Can you work these out from the model? Positions are in its coordinate system, mm. Face numbers are marked on the shaded views. Round coordinates to 2 decimals unless told otherwise and drop trailing zeros. Write each loop counter-clockwise with the first axis right and the second up, starting at its lowest first coordinate (ties: lowest second). Pieces come first, ordered by that corner, then holes.
Q1. We'd pull the mould along Z, two halves only. Please class the marked faces 1, 2, 3 and 4: +Z half, -Z half, draft (parallel to the pull), parting line (faces both ways), or undercut.
Q2. I'm going to push flat-ended pins straight in: pin 1 Ø5 at (y, z) = (-7, -2) entering from -X; pin 2 Ø5 at (x, z) = (13.5, 0) entering from +Y; pin 3 Ø1.5 at (y, z) = (-1.5, 9) entering from -X; pin 4 Ø1 at (x, y) = (-11.5, -4) entering from +Z. Where does each tip first touch, or does it pass through?
Q3. If we section it at B-B (y = -9.5): Please give me the cut outline in (x, z), plus the area to 3 significant figures.
Q4. If we section it at A-A (x = -5.5): Please give me the cut outline in (y, z).
Q5. Please list where these lines run through material, in increasing order: line 1 along Z through (x, y) = (13.5, -4); line 2 along Z through (x, y) = (-13, -10.5); line 3 along X through (y, z) = (-11, 1.5).
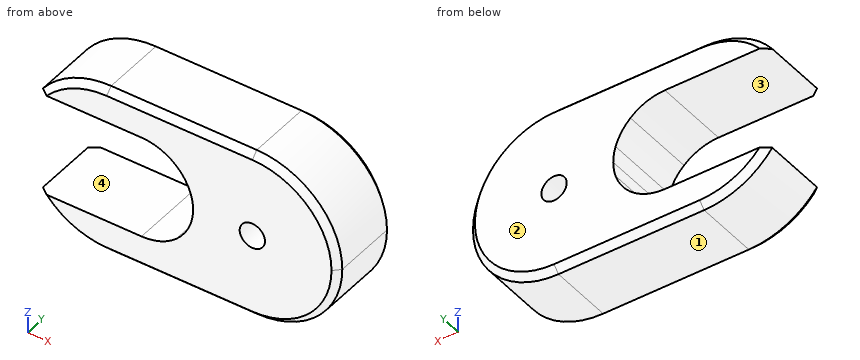
from build123d import *

# Parameters (mm, degrees)
F0_R     = 2
F1_DEPTH = 12
F2_SIZE  = 1


with BuildPart() as f1:
    # F0 (on Front) → F1 (new body)
    with BuildSketch(Plane.XZ):
        with BuildLine():
            ThreePointArc((-9.5, -13.5), (-2.9124896759, -11.7836627468), (2, -7.0710678119))
            ThreePointArc((2, -7.0710678119), (1.7096518051, -6.5755371981), (1.4406428571, -6.0681055776))
            ThreePointArc((1.4406428571, -6.0681055776), (-1.087317427, -7.6117527698), (-4, -8.15))
            Line((-4, -8.15), (-20.2623185234, -8.15))
            ThreePointArc((-20.2623185234, -8.15), (-15.5093676872, -12.0887344251), (-9.5, -13.5))
        make_face()
        with BuildLine():
            Line((-9.5, -13.5), (13.5, -13.5))
            ThreePointArc((13.5, -13.5), (6.9124896759, -11.7836627468), (2, -7.0710678119))
            ThreePointArc((2, -7.0710678119), (-2.9124896759, -11.7836627468), (-9.5, -13.5))
        make_face()
        with BuildLine():
            ThreePointArc((1.4406428571, 6.0681055776), (1.7096518051, 6.5755371981), (2, 7.0710678119))
            ThreePointArc((2, 7.0710678119), (-2.9124896759, 11.7836627468), (-9.5, 13.5))
            ThreePointArc((-9.5, 13.5), (-15.5093676872, 12.0887344251), (-20.2623185234, 8.15))
            Line((-20.2623185234, 8.15), (-4, 8.15))
            ThreePointArc((-4, 8.15), (-1.087317427, 7.6117527698), (1.4406428571, 6.0681055776))
        make_face()
        with BuildLine():
            ThreePointArc((3.7797727273, 2.4285049541), (3.1054603873, 4.8324288328), (2, 7.0710678119))
            ThreePointArc((2, 7.0710678119), (1.7096518051, 6.5755371981), (1.4406428571, 6.0681055776))
            ThreePointArc((1.4406428571, 6.0681055776), (2.8561301206, 4.4063567456), (3.7797727273, 2.4285049541))
        make_face()
        with BuildLine():
            ThreePointArc((2, 7.0710678119), (6.9124896759, 11.7836627468), (13.5, 13.5))
            Line((13.5, 13.5), (-9.5, 13.5))
            ThreePointArc((-9.5, 13.5), (-2.9124896759, 11.7836627468), (2, 7.0710678119))
        make_face()
        with BuildLine():
            ThreePointArc((13.5, -13.5), (23.045941546, -9.545941546), (27, 0))
            ThreePointArc((27, 0), (23.045941546, 9.545941546), (13.5, 13.5))
            ThreePointArc((13.5, 13.5), (6.9124896759, 11.7836627468), (2, 7.0710678119))
            ThreePointArc((2, 7.0710678119), (3.1054603873, 4.8324288328), (3.7797727273, 2.4285049541))
            ThreePointArc((3.7797727273, 2.4285049541), (4.0569115586, 1.2282817822), (4.15, 0))
            ThreePointArc((4.15, 0), (4.0569115586, -1.2282817822), (3.7797727273, -2.4285049541))
            ThreePointArc((3.7797727273, -2.4285049541), (3.1054603873, -4.8324288328), (2, -7.0710678119))
            ThreePointArc((2, -7.0710678119), (6.9124896759, -11.7836627468), (13.5, -13.5))
        make_face()
        with Locations((13.5, 0)):
            Circle(F0_R, mode=Mode.SUBTRACT)
        with BuildLine():
            ThreePointArc((1.4406428571, -6.0681055776), (1.7096518051, -6.5755371981), (2, -7.0710678119))
            ThreePointArc((2, -7.0710678119), (3.1054603873, -4.8324288328), (3.7797727273, -2.4285049541))
            ThreePointArc((3.7797727273, -2.4285049541), (2.8561301206, -4.4063567456), (1.4406428571, -6.0681055776))
        make_face()
    extrude(amount=F1_DEPTH)

    # F2
    f2_edges = [f1.edges().sort_by_distance(p)[0] for p in [
        (27, -12, 0),
        (27, 0, 0),
        (-15.509368, 0, -12.088734),
        (-15.509368, -12, -12.088734),
        (2, 0, -13.5),
        (2, -12, -13.5),
        (2, 0, 13.5),
        (2, -12, 13.5),
        (-15.509368, 0, 12.088734),
        (-15.509368, -12, 12.088734),
    ]]
    chamfer(f2_edges, length=F2_SIZE)


solid = f1.part
A:
1. face 1: -Z half
1. face 2: draft
1. face 3: undercut
1. face 4: undercut
2. pin 1: stops at x = 2.8
2. pin 2: stops at y = 0
2. pin 3: stops at x = -20.19
2. pin 4: stops at z = 13.42
3. outline: (-20.26, -8.15) arc R13.5 ccw to (-9.5, -13.5) - (13.5, -13.5) arc R13.5 ccw to (13.5, 13.5) - (-9.5, 13.5) arc R13.5 ccw to (-20.26, 8.15) - (-4, 8.15) arc R8.15 cw to (-4, -8.15) - close; hole circle Ø4 at (13.5, 0)
3. area: 781 mm2
4. outline: (-12, -12.5) - (-11, -13.5) - (-1, -13.5) - (0, -12.5) - (0, -8.15) - (-12, -8.15) - close; (-12, 8.15) - (0, 8.15) - (0, 12.5) - (-1, 13.5) - (-11, 13.5) - (-12, 12.5) - close
5. line 1: z = -13.5 to -2, 2 to 13.5
5. line 2: z = -13.04 to -8.15, 8.15 to 13.04
5. line 3: x = 4.01 to 12.18, 14.82 to 26.92
